The listing builds one solid part. Answer for the finished solid, in the listing's coordinates (mm). A direction names the side the tool comes from. Give positions to 0.01 mm unless a question says otherwise; leave off trailing zeros. Write each loop counter-clockwise with the first axis right and the second up, starting at its lowest first coordinate (ties: lowest second). Pieces come first, ordered by that corner, then holes.
Autodesk Inventor part; units mm, degrees
ref_plane "YZ Plane" through (0, 0, 0) normal (1, 0, 0) x (0, 1, 0)
ref_plane "XZ Plane" through (0, 0, 0) normal (0, 1, 0) x (-1, 0, 0)
ref_plane "XY Plane" through (0, 0, 0) normal (0, 0, 1) x (1, 0, 0)
sketch "Szkic1" plane through (0, 0, 0) normal (0, 0, 1) x (1, 0, 0)
  circle A0 centre (0, 0) radius 9
  dimension "d0" = 18
extrude "Wyciągnięcie proste1" add sketch "Szkic1" along normal mid plane 90
sketch "Szkic2" plane through (0, 0, 45) normal (0, 0, 1) x (1, 0, 0)
  circle A0 centre (0, 0) radius 9
  line L0 (-4.9749, 7.5) -> (4.9749, 7.5)
  line L1 (-6.5383, 2.5) -> (6.5383, 2.5)
  line L2 (-6.5, -2.5981) -> (-6.5, -6.2249)
  line L3 (6.5, -2.5981) -> (6.5, -6.2249)
  line L4 (0, 0) -> (0, -2.0526) construction
  arc A1 (-6.5383, 2.5) -> (-6.5, -2.5981) centre (0, 0) ccw
  arc A2 (6.5, -2.5981) -> (6.5383, 2.5) centre (0, 0) ccw
  arc A3 (-6.5, -6.2249) -> (6.5, -6.2249) centre (0, 0) ccw
  arc A4 (4.9749, 7.5) -> (-4.9749, 7.5) centre (0, 0) ccw
  dimension "d3" = 1.5
  dimension "d5" = 5
  dimension "d9" = 2
  dimension "d22" = 13
extrude "Wyciągnięcie proste2" cut sketch "Szkic2" against normal up to next contours L0 A0 | A0 L2 A1 L1 A2 L3
sketch "Szkic3" plane through (-4.9749, 7.5, 45) normal (0, 1, 0) x (1, 0, 0)
  line L0 (9.9499, 0) -> (0, 0)
  point P0 (4.9749, 45)
  point P1 (4.9749, 20)
  point P2 (4.9749, 50)
  point P3 (4.9749, 80)
  dimension "d12" = 20
  dimension "d13" = 30
  dimension "d14" = 30
hole "Otwór1" at (0, 7.5, 25) at (0, 7.5, -5) at (0, 7.5, -35) direction (0, -1, 0) diameter 6 end through all
properties part number "Pasek_reulacji" material "Stal nierdzewna"
Item 1: A cutting plane is placed at C-C, the plane z = 25. Give the vertices of the cut face in (x, y), plus the area to 3 significant figures.
Conclusion:
outline: (-6.54, 2.5) - (-3, 2.5) - (-3, 7.5) - (-4.97, 7.5) arc R9 ccw to (-6.5, -6.22) - (-6.5, -2.6) arc R7 cw to start; (3, 2.5) - (6.54, 2.5) arc R7 cw to (6.5, -2.6) - (6.5, -6.22) arc R9 ccw to (4.97, 7.5) - (3, 7.5) - close
area: 72.5 mm2
Item 2: A cutting plane is placed at B-B, the plane y = -1.5. Give the vertices of the cut face in (x, z), plus the area to 3 significant figures.
Conclusion:
outline: (-8.87, -45) - (-6.84, -45) - (-6.84, 45) - (-8.87, 45) - close; (6.84, -45) - (8.87, -45) - (8.87, 45) - (6.84, 45) - close
area: 367 mm2
Item 3: Consider probe 1 along Z at (x, y) = (0, 4.7); probe 2 along Y at (x, z) = (4, 3); probe 3 along X at (y, z) = (4.85, -35). Determine where each line is inside the solid, lowest interval first.
Conclusion:
probe 1: z = -45 to -38, -32 to -8, -2 to 22, 28 to 45
probe 2: y = 2.5 to 7.5
probe 3: x = -7.58 to -3, 3 to 7.58
Item 4: Each of these flat-tipped pins is pushed along its axis until it touches: P1, Ø1.5, axis at x = -4, z = -27.5, coming from the -Y side; P2, Ø5.5, axis at x = 0, z = -5, coming from the +Y side; P3, Ø3, axis at y = -4, z = -14, coming from the -X side; P4, Ø2, axis at y = 2, z = 19.5, coming from the -X side. Where does it stop, or does it pass through?
Conclusion:
P1: stops at y = 2.5
P2: passes through
P3: stops at x = -8.65
P4: stops at x = -8.94
Item 5: Determine the mould class of faces 3 (the face through (7, 0, 1)), 4 (the face through (0, 4, 45)), 5 (the face through (0, 7.5, 1)), 6 (the face through (-7, 0, 1)) for opening direction Y: pulls with the +Y half, pulls with the -Y half, needs draft (parallel to the pull), parting line crosses it, or undercut.
Conclusion:
face 3: undercut
face 4: needs draft
face 5: pulls with the +Y half
face 6: undercut
Item 6: Which of the six approach directions +Z, -Z, +X, -X, +Y, -Y give full straight-line access (tool end or side, diameter ignored) to faces 1 (the face through (-6.5, -4, 1)), 2 (the face through (0, 5, 22))?
Conclusion:
face 1: +Z, -Z, -Y
face 2: +Y, -Y
Item 7: A cutting plane is placed at D-D, the plane y = 5.5. Give the vertices of the cut face in (x, z).
Conclusion:
outline: (-7.12, -45) - (7.12, -45) - (7.12, 45) - (-7.12, 45) - close; hole circle Ø6 at (0, -35); hole circle Ø6 at (0, -5); hole circle Ø6 at (0, 25)
Item 8: A cutting plane is placed at A-A, the plane x = 0. Give the vertices of the cut face in (y, z), plus the area to 3 significant figures.
Conclusion:
outline: (2.5, -45) - (7.5, -45) - (7.5, -38) - (2.5, -38) - close; (2.5, -32) - (7.5, -32) - (7.5, -8) - (2.5, -8) - close; (2.5, -2) - (7.5, -2) - (7.5, 22) - (2.5, 22) - close; (2.5, 28) - (7.5, 28) - (7.5, 45) - (2.5, 45) - close
area: 360 mm2
